Source: CAD feature listing. Evaluate the final solid. Frame: model axes, mm. Face numbers are marked on the shaded views. A direction names the side the tool comes from. Coordinates: 2 decimals unless noted, no trailing zeros. Write each loop counter-clockwise with the first axis right and the second up, starting at its lowest first coordinate (ties: lowest second). Pieces come first, ordered by that corner, then holes. Notation, with made-up numbers: M 88,46.25 L 141,46.25 A24 cw 141,63.25 Z; hole C 43.25,63.25 d10. An arc over 180 degrees is marked long. One line per item, written item: value. Start each with the question number.
Item 1: Set-up query: the marked faces 4, 5 and 6. Return all of +Z, -Z, +X, -X, +Y, -Y with unobstructed straight access to the full face (end or side cutting, diameter ignored); none if empty.
Item 2: Pin query (flat end, axial travel): P1, Ø1, axis at x = 4.5, z = -1.5, coming from the -Y side. Return the tip coordinate at first contact, or that it passes through.
Item 3: Cut plane C-C, the plane x = -2.75. Output: boundary loops of the cut face in (y, z).
Item 4: Cut plane D-D, the plane y = -2. Output: boundary loops of the cut face in (x, z).
Item 5: Mould query, pull axis X, two halves, no side actions, for the marked faces 1, 2 and 3. Classes: released by +X, released by -X, zero draft, split by the parting line, or undercut.
Item 6: Cut plane A-A, the plane x = -11.25. Output: boundary loops of the cut face in (y, z), then the cut area to 3 significant figures.
Item 7: Cut plane B-B, the plane y = -6. Output: boundary loops of the cut face in (x, z).
Item 8: Ray query, L1, parallel to Y at x = 10.5, z = 2.15; L2, parallel to X at y = -10.25, z = 1.8; L3, parallel to X at y = 11, z = 2.35. Return the intervals inside material, ascending. Write a range as from..to.
```python
from build123d import *

# Parameters (mm, degrees)
SKETCH1_R           = 14
BOSS_EXTRUDE1_DEPTH = 2.5
CUT_EXTRUDE1_START  = 21.420577857
CUT_EXTRUDE1_DEPTH  = 26.420577857
FILLET1_R           = 0.25
CIRPATTERN1_COUNT   = 12
FILLET2_R           = 0.6
FILLET3_R           = 0.6
FILLET4_R           = 0.6
FILLET5_R           = 0.6


with BuildPart() as part:
    # Sketch1 → Boss-Extrude1 (new, symmetric)
    with BuildSketch(Plane.XY):
        Circle(SKETCH1_R)
    extrude(amount=BOSS_EXTRUDE1_DEPTH, both=True)

    # Sketch2 → Cut-Extrude1 (cut)
    with BuildSketch(Plane.XY.offset(2.5).offset(CUT_EXTRUDE1_START)):
        with BuildLine():
            ThreePointArc((-0.430438648, 9.490243546), (-0.222226767, 11.808448469), (0.596346311, 13.987293201))
            ThreePointArc((0.596346311, 13.987293201), (-1.425202617, 13.927268128), (-3.417009435, 13.576599225))
            ThreePointArc((-3.417009435, 13.576599225), (-2.174093588, 11.608710395), (-1.50066187, 9.380725662))
            ThreePointArc((-1.50066187, 9.380725662), (-0.967101776, 9.450646229), (-0.430438648, 9.490243546))
        make_face()
    cut_extrude1 = extrude(amount=-CUT_EXTRUDE1_DEPTH, mode=Mode.SUBTRACT)

    # Fillet1
    fillet1_edges = [part.edges().sort_by_distance(p)[0] for p in [
        (-1.50066187, 9.380725662, 0),
        (-0.430438648, 9.490243546, 0),
    ]]
    fillet(fillet1_edges, radius=FILLET1_R)

    # CirPattern1: Cut-Extrude1 ×12 about axis
    cirpattern1_axis = Axis((0, 0, 2.5), (0, 0, 1))
    for i in range(1, CIRPATTERN1_COUNT):
        add(cut_extrude1.rotate(cirpattern1_axis, i * 360 / CIRPATTERN1_COUNT), mode=Mode.SUBTRACT)

    # Fillet2
    # the kernel refuses this fillet: 0.6 mm, written as the material it adds along each edge
    with BuildSketch(Plane(origin=(-5.989974133, 7.373615794, 2.5), x_dir=(-0.6546840177965881, 0.7559026636027397, 0), z_dir=(0, 0, -1))) as fillet2_piece_1:
        with BuildLine():
            CenterArc((0.564611753, 0.599701652), FILLET2_R, 185.108089024, 83.084978973)
            ThreePointArc((-0.03300535, 0.546280701), (-0.012568085, 0.273378072), (0, 0))
            ThreePointArc((0, 0), (0.272846371, 0.004302723), (0.545692742, 0))
        make_face()
    extrude(amount=5)
    with BuildSketch(Plane(origin=(-5.117892577, 8.003572675, 2.5), x_dir=(-0.8266142951027914, -0.5627688754113143, 0), z_dir=(0, 0, -1))) as fillet2_piece_2:
        with BuildLine():
            CenterArc((0.564559284, 0.599751046), FILLET2_R, 185.264442517, 83.084978973)
            ThreePointArc((-0.032909815, 0.54469947), (-0.012160017, 0.272609225), (0, 0))
            ThreePointArc((0, 0), (0.273638428, 0.003941765), (0.547276857, 0))
        make_face()
    extrude(amount=5)

    # Fillet3
    # the kernel refuses this fillet: 0.6 mm, written as the material it adds along each edge
    with BuildSketch(Plane(origin=(-8.874277665, 3.390751529, 2.5), x_dir=(-0.9449243226648774, 0.3272889005700054, 0), z_dir=(0, 0, -1))) as fillet3_piece_1:
        with BuildLine():
            CenterArc((0.564611753, 0.599701652), FILLET3_R, 185.108089024, 83.084978973)
            ThreePointArc((-0.03300535, 0.546280701), (-0.012568085, 0.273378072), (0, 0))
            ThreePointArc((0, 0), (0.272846371, 0.004302723), (0.545692742, 0))
        make_face()
    extrude(amount=5)
    with BuildSketch(Plane(origin=(-8.434011323, 4.372350969, 2.5), x_dir=(-0.4344845409847307, -0.9006792901167916, 0), z_dir=(0, 0, -1))) as fillet3_piece_2:
        with BuildLine():
            CenterArc((0.564559284, 0.599751046), FILLET3_R, 185.264442517, 83.084978973)
            ThreePointArc((-0.032909815, 0.54469947), (-0.012160017, 0.272609225), (0, 0))
            ThreePointArc((0, 0), (0.273638428, 0.003941765), (0.547276857, 0))
        make_face()
    extrude(amount=5)

    # Fillet4
    # the kernel refuses this fillet: 0.6 mm, written as the material it adds along each edge
    with BuildSketch(Plane(origin=(-9.380725662, -1.50066187, 2.5), x_dir=(-0.9819729183665902, -0.18902165906213533, 0), z_dir=(0, 0, -1))) as fillet4_piece_1:
        with BuildLine():
            CenterArc((0.564611753, 0.599701652), FILLET4_R, 185.108089024, 83.084978973)
            ThreePointArc((-0.03300535, 0.546280701), (-0.012568085, 0.273378072), (0, 0))
            ThreePointArc((0, 0), (0.272846371, 0.004302723), (0.545692742, 0))
        make_face()
    extrude(amount=5)
    with BuildSketch(Plane(origin=(-9.490243546, -0.430438648, 2.5), x_dir=(0.07406499501400296, -0.997253416396041, 0), z_dir=(0, 0, -1))) as fillet4_piece_2:
        with BuildLine():
            CenterArc((0.564559284, 0.599751046), FILLET4_R, 185.264442517, 83.084978973)
            ThreePointArc((-0.032909815, 0.54469947), (-0.012160017, 0.272609225), (0, 0))
            ThreePointArc((0, 0), (0.273638428, 0.003941765), (0.547276857, 0))
        make_face()
    extrude(amount=5)

    # Fillet5
    # the kernel refuses this fillet: 0.6 mm, written as the material it adds along each edge
    with BuildSketch(Plane(origin=(-7.373615794, -5.989974133, 2.5), x_dir=(-0.7559026636027405, -0.6546840177965871, 0), z_dir=(0, 0, -1))) as fillet5_piece_1:
        with BuildLine():
            CenterArc((0.564611753, 0.599701652), FILLET5_R, 185.108089024, 83.084978973)
            ThreePointArc((-0.03300535, 0.546280701), (-0.012568085, 0.273378072), (0, 0))
            ThreePointArc((0, 0), (0.272846371, 0.004302723), (0.545692742, 0))
        make_face()
    extrude(amount=5)
    with BuildSketch(Plane(origin=(-8.003572675, -5.117892577, 2.5), x_dir=(0.562768875411312, -0.8266142951027928, 0), z_dir=(0, 0, -1))) as fillet5_piece_2:
        with BuildLine():
            CenterArc((0.564559284, 0.599751046), FILLET5_R, 185.264442517, 83.084978973)
            ThreePointArc((-0.032909815, 0.54469947), (-0.012160017, 0.272609225), (0, 0))
            ThreePointArc((0, 0), (0.273638428, 0.003941765), (0.547276857, 0))
        make_face()
    extrude(amount=5)


solid = part.part
```
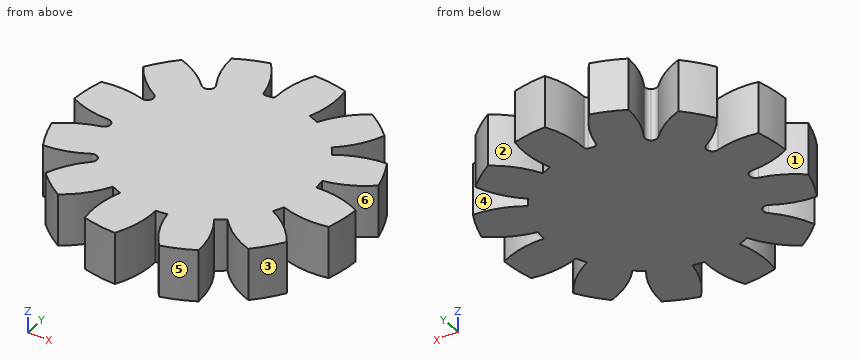
From the geometry:
1. face 4: +Z, -Z
1. face 5: +Z, -Z, +X, -Y
1. face 6: +Z, -Z, +X
2. P1: stops at y = -13.42
3. outline: M -13.73,-2.5 L 12.67,-2.5 L 12.67,2.5 L -13.73,2.5 Z
4. outline: M -11.2,-2.5 L 13.86,-2.5 L 13.86,2.5 L -11.2,2.5 Z
5. face 1: released by -X
5. face 2: undercut
5. face 3: released by +X
6. outline: M -6.36,-2.5 L -2.02,-2.5 L -2.02,2.5 L -6.36,2.5 Z; M -0.33,-2.5 L 3.93,-2.5 L 3.93,2.5 L -0.33,2.5 Z; M 6.7,-2.5 L 8.33,-2.5 L 8.33,2.5 L 6.7,2.5 Z
6. area: 51.2 mm²
7. outline: M -12.65,-2.5 L -9.82,-2.5 L -9.82,2.5 L -12.65,2.5 Z; M -7.6,-2.5 L 10.63,-2.5 L 10.63,2.5 L -7.6,2.5 Z
8. L1: y = -9.26..-5.87, -3.84..0.42, 1.76..6.21
8. L2: x = -9.54..-5.63, -3.79..0.43, 1.69..6.14
8. L3: x = -6.32..-1.92, -0.37..3.91, 6.4..8.66
